```python
from build123d import *

# Parameters (mm, degrees)
CHAMFER1_SIZE = 1.5


with BuildPart() as part:
    # Sketch1 → Revolve1 (revolve)
    with BuildSketch(Plane.XY, mode=Mode.PRIVATE) as revolve1_sk:
        Polygon((0, 32.5), (-25.5, 32.5), (-25.5, 30), (-54.5, 30), (-54.5, 29), (-94.5, 29), (-94.5, 27.5), (-97.5, 27.5), (-97.5, 26.5), (-98.5, 26.5), (-98.5, 27.5), (-126.5, 27.5), (-126.5, 22.5), (0, 22.5), align=None)
    revolve1 = revolve(revolve1_sk.sketch.rotate(Axis((0, 0, 0), (1, 0, 0)), 90), axis=Axis((0, 0, 0), (1, 0, 0)))

    # Mirror1: Revolve1 across plane
    add(revolve1.mirror(Plane(origin=(0, 0, 0), x_dir=(0, 0, 1), z_dir=(1, 0, 0))))

    # Chamfer1
    chamfer1_edges = [part.edges().sort_by_distance(p)[0] for p in [
        (-126.5, 0, -27.5),
        (126.5, 0, -27.5),
    ]]
    chamfer(chamfer1_edges, length=CHAMFER1_SIZE)


solid = part.part
```
Source: CAD feature listing. Evaluate the final solid. Frame: model axes, mm. A direction names the side the tool comes from. Round coordinates to 2 decimals unless told otherwise and drop trailing zeros. Loops run counter-clockwise (first coordinate to the right, second up) from the corner with the lowest first, then second, coordinate; pieces in that order, holes last. Notation, with made-up numbers: M 30.5,-19.75 L 55.5,-19.75 A16 cw 55.5,8.25 Z; hole C 28,-16 d6. An arc over 180 degrees is marked long. Put each result on its own line as item: value.
(1) Pull-direction query (X, two-part tool) for faces 1 (the face through (111.936, 24.397, 12.69)), 2 (the face through (-98.007, -26.274, -3.45)), 3 (the face through (-97.5, -23, -14)), 4 (the face through (-54.5, -25, -16)); classes: released by +X, released by -X, zero draft, split by the parting line, or undercut.
Solutions:
face 1: zero draft
face 2: undercut
face 3: undercut
face 4: released by -X
(2) Section B-B, the plane x = -18. Return loops of the section in (y, z), and give its area (3 significant figures).
Solutions:
outline: C 0,0 d65; hole C 0,0 d45
area: 1,730 mm²
(3) Access query for faces 5 (the face through (25.5, 29, 9)), 6 (the face through (-98.5, -14, 23)), 7 (the face through (126.5, -19.4, -11.7)), 8 (the face through (-40.203, -25.296, 16.128)). Directions: +Z, -Z, +X, -X, +Y, -Y. A direction counts if a zero-diameter tool reaches every point of the face in a straight line with its end or side. Return the directions, or none.
Solutions:
face 5: +X
face 6: none
face 7: +Z, -Z, +X, +Y, -Y
face 8: -X
(4) First-contact query: pin 1 (2 mm diameter, centred on x = -9, y = -13, fed in from +Z); pin 2 (4 mm diameter, centred on y = 25.5, z = -20, fed in from +X); pin 3 (2 mm diameter, centred on x = 99, z = 11, fed in from +Y). Flat tips, straight axial feed; report the tip coordinate or a pass-through.
Solutions:
pin 1: z = 30.2
pin 2: x = 25.5
pin 3: y = 25.62
(5) Section A-A, the plane x = -44.5. Return loops of the section in (y, z), and give its area (3 significant figures).
Solutions:
outline: C 0,0 d60; hole C 0,0 d45
area: 1,240 mm²
(6) Ray query, line 1 (X direction, y = -28, z = -1.5); line 2 (X direction, y = -8.5, z = -29); line 3 (Y direction, x = 56, z = 0). Return the intervals inside material, ascending. Write a range as [from, to].
Solutions:
line 1: [-94.5, 94.5]
line 2: [-25.5, 25.5]
line 3: [-29, -22.5], [22.5, 29]
